Verification items for the finished model (mm, model axes). A direction names the side the tool comes from. Give positions to 0.01 mm unless a question says otherwise; leave off trailing zeros. Order: outer loops, then holes, each group sorted by start corner. A loop starts at its lowest first (then second) coordinate and runs counter-clockwise, first axis right, second up.
from build123d import *

# Parameters (mm, degrees)
F1_DEPTH = 82.55
F3_DEPTH = 25.4
F5_DEPTH = 66.676
F6_R     = 3.175
F7_R     = 6.35


with BuildPart() as f1:
    # F0 (on Front) → F1 (new body)
    with BuildSketch(Plane.XZ):
        Polygon((0, 66.675), (0, 0), (200.025, 0), (200.025, 19.05), (93.121408, 19.05), (93.121408, 63.413289), (83.596408, 63.413289), (54.240717, 34.057599), (54.240717, 28.052471), (41.540717, 28.052471), (41.802945, 34.397055), (9.525, 66.675), align=None)
    extrude(amount=F1_DEPTH)

    # F2 (on Top) → F3 (join)
    with BuildSketch(Plane.XY):
        with BuildLine():
            Line((168.175783, -22.225), (123.725783, -22.225))
            ThreePointArc((123.725783, -22.225), (104.675783, -41.275), (123.725783, -60.325))
            Line((123.725783, -60.325), (168.175783, -60.325))
            ThreePointArc((168.175783, -60.325), (187.225783, -41.275), (168.175783, -22.225))
        make_face()
    extrude(amount=F3_DEPTH)

    # F4 (on Top) → F5 (cut, through all)
    with BuildSketch(Plane.XY):
        with BuildLine():
            ThreePointArc((124.727895, -31.75), (115.202895, -41.275), (124.727895, -50.8))
            Line((124.727895, -50.8), (169.177895, -50.8))
            ThreePointArc((169.177895, -50.8), (178.702895, -41.275), (169.177895, -31.75))
            Line((169.177895, -31.75), (124.727895, -31.75))
        make_face()
    extrude(amount=F5_DEPTH, mode=Mode.SUBTRACT)

    # F6
    f6_edges = [f1.edges().sort_by_distance(p)[0] for p in [
        (145.950783, -60.325, 19.05),
    ]]
    fillet(f6_edges, radius=F6_R)

    # F7
    f7_edges = [f1.edges().sort_by_distance(p)[0] for p in [
        (93.121408, -41.275, 19.05),
    ]]
    fillet(f7_edges, radius=F7_R)


solid = f1.part
(1) Section check D-D, the plane x = 26.5. Enter the section's corners in (y, z), then the cut area to 3 significant figures.
Solved:
outline: (-82.55, 0) - (0, 0) - (0, 49.7) - (-82.55, 49.7) - close
area: 4,100 mm2
(2) Section check A-A, the plane z = 10.5. Enter the section's corners in (x, y) (3 decimals), then the cut area to 3 significant figures.
Solved:
outline: (0, -82.55) - (200.025, -82.55) - (200.025, 0) - (0, 0) - close; hole (124.728, -50.8) - (169.178, -50.8) arc R9.525 ccw to (169.178, -31.75) - (124.728, -31.75) arc R9.525 ccw to start
area: 15,400 mm2
(3) Section check C-C, the plane z = 54. Enter the section's corners in (x, y), then the cut area to 3 significant figures.
Solved:
outline: (0, -82.55) - (22.2, -82.55) - (22.2, 0) - (0, 0) - close; (74.18, -82.55) - (93.12, -82.55) - (93.12, 0) - (74.18, 0) - close
area: 3,400 mm2
(4) Scan lines: line 1 (X direction, y = -41, z = 18) (3 decimals); line 2 (Y direction, x = 162, z = 13.5); line 3 (Z direction, x = 106, y = -12.5). Record each from-to range of solid material in increasing order.
Solved:
line 1: x = 0 to 115.207, 178.699 to 200.025
line 2: y = -82.55 to -50.8, -31.75 to 0
line 3: z = 0 to 19.05
(5) Release check for a two-part mould opening along X. For faces 1 (the flat face through (0, -41, 34)), 2 (the flat face through (5, -41, 66.675)), 3 (the cylindrical face through (104.68, -40.86, 23.79)) record: pulls with the +X half, pulls with the -X half, needs draft (parallel to the pull), parting line crosses it, or undercut.
Solved:
face 1: pulls with the -X half
face 2: needs draft
face 3: undercut
(6) Section check B-B, the plane y = -17. Enter the section's corners in (x, z) (3 decimals).
Solved:
outline: (0, 0) - (200.025, 0) - (200.025, 19.05) - (99.471, 19.05) arc R6.35 cw to (93.121, 25.4) - (93.121, 63.413) - (83.596, 63.413) - (54.241, 34.058) - (54.241, 28.052) - (41.541, 28.052) - (41.803, 34.397) - (9.525, 66.675) - (0, 66.675) - close
(7) Go/stop test with flat-tipped pins: pin 1 (3.5 mm diameter, centred on x = 141.5, z = 24, fed in from -Y) (3 decimals); pin 2 (19 mm diameter, centred on y = -53.5, z = 44, fed in from +X); pin 3 (7.5 mm diameter, centred on x = 86.5, y = -38, fed in from +Z); pin 4 (12 mm diameter, centred on x = 177, z = 33, fed in from -Y). Record where each tip stops, or that it passes through.
Solved:
pin 1: stops at y = -60.325
pin 2: stops at x = 93.12
pin 3: stops at z = 63.41
pin 4: passes through
(8) Set-up check for faces 4 (the flat face through (88, -41, 63.413)), 5 (the cylindrical face through (187.22, -41.69, 23.79)), 6 (the flat face through (76, -82.55, 19)), 7 (the flat face through (147, -31.75, 13)), 8 (the flat face through (54.241, -41, 31)): record each of +Z, -Z, +X, -X, +Y, -Y from which the full face is reachable in a straight line by a thin tool's end or side.
Solved:
face 4: +Z, +X, +Y, -Y
face 5: +Z, +X
face 6: +Z, -Z, +X, -X, -Y
face 7: +Z, -Z
face 8: +Z, +Y, -Y
